Could you check a few things on this drawing? It's one solid part, dimensions in mm from its lowest x, y, z. A direction names the side the tool comes from. Coordinates: 2 decimals unless noted, no trailing zeros. Loops run counter-clockwise (first coordinate to the right, second up) from the corner with the lowest first, then second, coordinate; pieces in that order, holes last. Notation, with made-up numbers: M 56.5,24.5 L 86.5,24.5 A14 ccw 86.5,33.5 Z; hole C -11.5,59.25 d8. An arc over 180 degrees is marked long. Use one line per item in the form item = value. Start each with the question number.
(1) Imagine slicing it at B-B, the plane z = 6. Please give me the cut outline in (x, y), and give its area (3 significant figures).
(2) Thinking about a two-plate mould opening in X: for the marked faces 1, 2 and 3, which applies, +X half, -X half, draft (parallel to the pull), parting line (faces both ways), or undercut?
(3) Imagine slicing it at C-C, the plane x = 13.5. Please give me the cut outline in (y, z).
(4) Imagine slicing it at A-A, the plane y = 32.5. Please give me the cut outline in (x, z), and give its area (3 significant figures).
(5) Will these pins go through, and if not, where does the flat tip stop? P1, Ø4, axis at x = 30, y = 11, coming from the +Z side; P2, Ø8, axis at x = 15, y = 37, coming from the -Z side; P3, Ø1.5, axis at x = 45, z = 9, coming from the -Y side; P4, Ø3.5, axis at x = 13, z = 8, coming from the -Y side.
(6) Imagine slicing it at D-D, the plane y = 4. Please give me the cut outline in (x, z), and give its area (3 significant figures).
(7) On a 3-axis mill with a long thin cutter (end or side, diameter ignored), from which of +Z, -Z, +X, -X, +Y, -Y can I reach the whole of each face in a straight line? I mean the marked faces 4, 5 and 6. Say none if no direction works.
(8) Please list where these lines run through material, in increasing order: L1, parallel to Y at x = 11.55, z = 6; L2, parallel to Z at x = 24, y = 33.
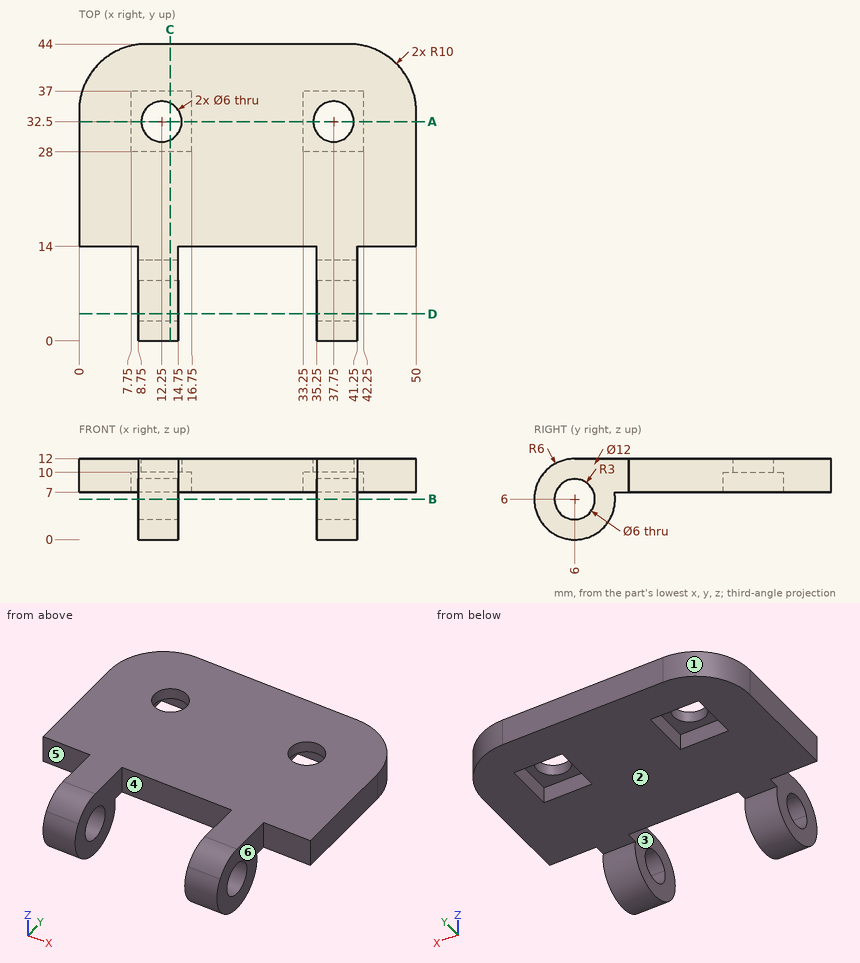
Answer:
q1.outline = M 8.75,0 L 14.75,0 L 14.75,3 L 8.75,3 Z; M 8.75,9 L 14.75,9 L 14.75,12 L 8.75,12 Z; M 35.25,0 L 41.25,0 L 41.25,3 L 35.25,3 Z; M 35.25,9 L 41.25,9 L 41.25,12 L 35.25,12 Z
q1.area = 72.0 mm²
q2.face_1 = -X half
q2.face_2 = draft
q2.face_3 = undercut
q3.outline = M 6,12 A6 ccw long 11.92,7 L 28,7 L 28,10 L 29.77,10 L 29.77,12 Z; M 35.23,10 L 37,10 L 37,7 L 44,7 L 44,12 L 35.23,12 Z; hole C 6,6 d6
q4.outline = M 0,7 L 7.75,7 L 7.75,10 L 9.25,10 L 9.25,12 L 0,12 Z; M 15.25,10 L 16.75,10 L 16.75,7 L 33.25,7 L 33.25,10 L 34.75,10 L 34.75,12 L 15.25,12 Z; M 40.75,10 L 42.25,10 L 42.25,7 L 50,7 L 50,12 L 40.75,12 Z
q4.area = 172 mm²
q5.P1 = through
q5.P2 = 7
q5.P3 = 14
q5.P4 = 0.01
q6.outline = M 8.75,0.34 L 14.75,0.34 L 14.75,3.76 L 8.75,3.76 Z; M 8.75,8.24 L 14.75,8.24 L 14.75,11.66 L 8.75,11.66 Z; M 35.25,0.34 L 41.25,0.34 L 41.25,3.76 L 35.25,3.76 Z; M 35.25,8.24 L 41.25,8.24 L 41.25,11.66 L 35.25,11.66 Z
q6.area = 82.1 mm²
q7.face_4 = +Z, -Z, -Y
q7.face_5 = +Z, -Z, -X, -Y
q7.face_6 = +Z, -Z, +X, -Y
q8.L1 = 0 to 3, 9 to 12
q8.L2 = 7 to 12
